Can you work these out from the model? Positions are in its coordinate system, mm. Give positions to 0.01 mm unless a question says otherwise; leave off trailing zeros. Write each loop counter-clockwise with the first axis right and the second up, starting at its lowest first coordinate (ties: lowest second). Pieces come first, ordered by that corner, then holes. Notation, with made-up numbers: (-22.75, 76) -> (-10.75, 76) arc R6 cw to (-10.75, 83) -> close; hole circle Ø4 at (-5.75, -21). An arc over 180 degrees is marked (long way). One line per item, written item: value.
from build123d import *

# Parameters (mm, degrees)
F0_W      = 44.656470418
F0_H      = 33.8078811765
F1_DEPTH  = 16
F2_DEPTH  = 796
F3_DEPTH  = 196
F4_W      = 68.9578056335
F4_H      = 493.6993122101
F5_DEPTH  = 7
F6_DEPTH  = 9.7
F7_DEPTH  = 99.33
F8_DEPTH  = 99.33
F9_DEPTH  = 17.34
F10_DEPTH = 102.97
F11_W     = 35.2807044983
F11_H     = 492.0964837074
F12_DEPTH = 7
F13_DEPTH = 37.27
F14_DEPTH = 6.58
F15_DEPTH = 106.63
F16_DEPTH = 5.87
F17_DEPTH = 200
F18_DEPTH = 200
F19_DEPTH = 200
F20_DEPTH = 600
F21_DEPTH = 600
F22_DEPTH = 600
F23_DEPTH = 200
F24_DEPTH = 200
F25_DEPTH = 200
F26_DEPTH = 200
F27_DEPTH = 200
F28_DEPTH = 200
F29_R     = 3


with BuildPart() as f1:
    # F0 (on Front) → F1 (new body)
    with BuildSketch(Plane.XZ):
        with Locations((22.328235209, 16.9039405882)):
            Rectangle(F0_W, F0_H)
    extrude(amount=F1_DEPTH)

    # F2 (add): a face of the model
    f2_faces = [f1.faces().sort_by_distance(p)[0] for p in [
        (22.328235209, -8, 0),
    ]]
    extrude(f2_faces, amount=-F2_DEPTH)

    # F3 (add): a face of the model
    f3_faces = [f1.faces().sort_by_distance(p)[0] for p in [
        (0, -8, 398),
    ]]
    extrude(f3_faces, amount=-F3_DEPTH)

    # F4 (on face) → F5 (cut)
    with BuildSketch(Plane.XZ.offset(16)):
        with Locations((94.1769480705, 399.8196721077)):
            Rectangle(F4_W, F4_H)
    extrude(amount=-F5_DEPTH, mode=Mode.SUBTRACT)

    # F6 (cut): a face of the model
    f6_faces = [f1.faces().sort_by_distance(p)[0] for p in [
        (59.6980452538, -12.5, 399.8196721077),
    ]]
    extrude(f6_faces, amount=-F6_DEPTH, mode=Mode.SUBTRACT)

    # F7 (add): a face of the model
    f7_faces = [f1.faces().sort_by_distance(p)[0] for p in [
        (89.3269480705, -12.5, 646.6693282127),
    ]]
    extrude(f7_faces, amount=-F7_DEPTH)

    # F8 (cut): a face of the model
    f8_faces = [f1.faces().sort_by_distance(p)[0] for p in [
        (89.3269480705, -12.5, 646.6693282127),
    ]]
    extrude(f8_faces, amount=-F8_DEPTH, mode=Mode.SUBTRACT)

    # F9 (cut): a face of the model
    f9_faces = [f1.faces().sort_by_distance(p)[0] for p in [
        (128.6558508873, -12.5, 449.4846721077),
    ]]
    extrude(f9_faces, amount=-F9_DEPTH, mode=Mode.SUBTRACT)

    # F10 (cut): a face of the model
    f10_faces = [f1.faces().sort_by_distance(p)[0] for p in [
        (97.9969480705, -12.5, 152.9700160027),
    ]]
    extrude(f10_faces, amount=-F10_DEPTH, mode=Mode.SUBTRACT)

    # F11 (on face) → F12 (join)
    with BuildSketch(Plane.XZ.offset(9)):
        with Locations((91.7714834213, 432.6795041561)):
            Rectangle(F11_W, F11_H)
    extrude(amount=F12_DEPTH)

    # F13 (add): a face of the model
    f13_faces = [f1.faces().sort_by_distance(p)[0] for p in [
        (91.7714834213, -12.5, 678.7277460098),
    ]]
    extrude(f13_faces, amount=F13_DEPTH)

    # F14 (add): a face of the model
    f14_faces = [f1.faces().sort_by_distance(p)[0] for p in [
        (109.4118356705, -12.5, 451.3145041561),
    ]]
    extrude(f14_faces, amount=F14_DEPTH)

    # F15 (add): a face of the model
    f15_faces = [f1.faces().sort_by_distance(p)[0] for p in [
        (95.0614834213, -12.5, 186.6312623024),
    ]]
    extrude(f15_faces, amount=F15_DEPTH)

    # F16 (cut): a face of the model
    f16_faces = [f1.faces().sort_by_distance(p)[0] for p in [
        (74.1311311722, -12.5, 397.9995041561),
    ]]
    extrude(f16_faces, amount=-F16_DEPTH, mode=Mode.SUBTRACT)

    # F17 (add): a face of the model
    f17_faces = [f1.faces().sort_by_distance(p)[0] for p in [
        (196, -8, 398),
    ]]
    extrude(f17_faces, amount=F17_DEPTH)

    # F18 (cut): a face of the model
    f18_faces = [f1.faces().sort_by_distance(p)[0] for p in [
        (145.9958508873, -12.5, 397.9996721077),
    ]]
    extrude(f18_faces, amount=-F18_DEPTH, mode=Mode.SUBTRACT)

    # F19 (add): a face of the model
    f19_faces = [f1.faces().sort_by_distance(p)[0] for p in [
        (115.9918356705, -12.5, 397.9995041561),
    ]]
    extrude(f19_faces, amount=F19_DEPTH)

    # F20 (cut): a face of the model
    f20_faces = [f1.faces().sort_by_distance(p)[0] for p in [
        (197.9964834213, -12.5, 80.0012623024),
    ]]
    extrude(f20_faces, amount=-F20_DEPTH, mode=Mode.SUBTRACT)

    # F21 (add): a face of the model
    f21_faces = [f1.faces().sort_by_distance(p)[0] for p in [
        (197.9969480705, -12.5, 50.0000160027),
    ]]
    extrude(f21_faces, amount=F21_DEPTH)

    # F22 (cut): a face of the model
    f22_faces = [f1.faces().sort_by_distance(p)[0] for p in [
        (198, -8, 0),
    ]]
    extrude(f22_faces, amount=-F22_DEPTH, mode=Mode.SUBTRACT)

    # F23 (add): a face of the model
    f23_faces = [f1.faces().sort_by_distance(p)[0] for p in [
        (198, -8, 600),
    ]]
    extrude(f23_faces, amount=F23_DEPTH)

    # F24 (cut): a face of the model
    f24_faces = [f1.faces().sort_by_distance(p)[0] for p in [
        (197.9969480705, -12.5, 650.0000160027),
    ]]
    extrude(f24_faces, amount=-F24_DEPTH, mode=Mode.SUBTRACT)

    # F25 (add): a face of the model
    f25_faces = [f1.faces().sort_by_distance(p)[0] for p in [
        (197.9964834213, -12.5, 680.0012623024),
    ]]
    extrude(f25_faces, amount=F25_DEPTH)

    # F26 (add): a face of the model
    f26_faces = [f1.faces().sort_by_distance(p)[0] for p in [
        (198, -8, 796),
    ]]
    extrude(f26_faces, amount=F26_DEPTH)

    # F27 (cut): a face of the model
    f27_faces = [f1.faces().sort_by_distance(p)[0] for p in [
        (197.9969480705, -12.5, 745.9993282127),
    ]]
    extrude(f27_faces, amount=-F27_DEPTH, mode=Mode.SUBTRACT)

    # F28 (add): a face of the model
    f28_faces = [f1.faces().sort_by_distance(p)[0] for p in [
        (197.9964834213, -12.5, 715.9977460098),
    ]]
    extrude(f28_faces, amount=F28_DEPTH)

    # F29
    f29_edges = [f1.edges().sort_by_distance(p)[0] for p in [
        (0, -16, 698),
        (198, -16, 400),
        (396, -16, 698),
        (198, -16, 996),
        (197.996948, -16, 450.000016),
        (49.998045, -16, 697.999672),
        (197.996948, -16, 945.999328),
        (345.995851, -16, 697.999672),
        (197.996483, -16, 480.001262),
        (80.001131, -16, 697.999504),
        (197.996483, -16, 915.997746),
        (315.991836, -16, 697.999504),
    ]]
    fillet(f29_edges, radius=F29_R)


solid = f1.part
1) I need wall thicknesses on L1, parallel to Z at x = 189.5, y = -11; L2, parallel to X at y = -9.25, z = 584; L3, parallel to Z at x = 102, y = -15. Which ranges of each line are inside material? Lowest first, please.
Answer list:
L1: z = 400 to 450, 480 to 916, 946 to 996
L2: x = 0 to 50, 80 to 315.99, 346 to 396
L3: z = 400.76 to 449.24, 480.77 to 915.23, 946.76 to 995.24
2) Will this pin go through, and if not, where does the flat tip stop? pin 1 (12 mm diameter, centred on x = 323, z = 615.5, fed in from -Y).
Answer list:
pin 1: stops at y = -9
3) If we section it at B-B (x = 176): Write out the boundary of the cut face in (y, z), and give its area (3 significant figures).
Answer list:
outline: (-16, 403) arc R3 ccw to (-13, 400) -> (0, 400) -> (0, 996) -> (-13, 996) arc R3 ccw to (-16, 993) -> (-16, 949) arc R3 ccw to (-13, 946) -> (-9, 946) -> (-9, 916) -> (-13, 916) arc R3 ccw to (-16, 913) -> (-16, 483) arc R3 ccw to (-13, 480) -> (-9, 480) -> (-9, 450) -> (-13, 450) arc R3 ccw to (-16, 447) -> close
area: 9,100 mm^2
4) If we section it at A-A (z = 940): Write out the boundary of the cut face in (x, y).
Answer list:
outline: (0, -13) arc R3 ccw to (3, -16) -> (47, -16) arc R3 ccw to (50, -13) -> (50, -9) -> (346, -9) -> (346, -13) arc R3 ccw to (349, -16) -> (393, -16) arc R3 ccw to (396, -13) -> (396, 0) -> (0, 0) -> close
5) We'd pull the mould along Z, two halves only. Please class faces 1 (the face through (27, -16, 694)), 2 (the face through (195, -6, 400)), 3 (the face through (77, -9, 715)): released by +Z, released by -Z, zero draft, split by the parting line, or undercut.
Answer list:
face 1: zero draft
face 2: released by -Z
face 3: undercut
6) If we section it at D-D (x = 330.5): Write out the boundary of the cut face in (y, z), and give its area (3 significant figures).
Answer list:
outline: (-16, 403) arc R3 ccw to (-13, 400) -> (0, 400) -> (0, 996) -> (-13, 996) arc R3 ccw to (-16, 993) -> (-16, 949) arc R3 ccw to (-13, 946) -> (-9, 946) -> (-9, 450) -> (-13, 450) arc R3 ccw to (-16, 447) -> close
area: 6,060 mm^2
7) If we section it at C-C (z = 499.5): Write out the boundary of the cut face in (x, y).
Answer list:
outline: (0, -13) arc R3 ccw to (3, -16) -> (47, -16) arc R3 ccw to (50, -13) -> (50, -9) -> (80, -9) -> (80, -13) arc R3 ccw to (83, -16) -> (312.99, -16) arc R3 ccw to (315.99, -13) -> (315.99, -9) -> (346, -9) -> (346, -13) arc R3 ccw to (349, -16) -> (393, -16) arc R3 ccw to (396, -13) -> (396, 0) -> (0, 0) -> close
